Geometry: see drawing. Coordinates: mm, zero at the bounding-box minimum. Give positions to 0.01 mm unless a question says otherwise; leave off trailing zeros.
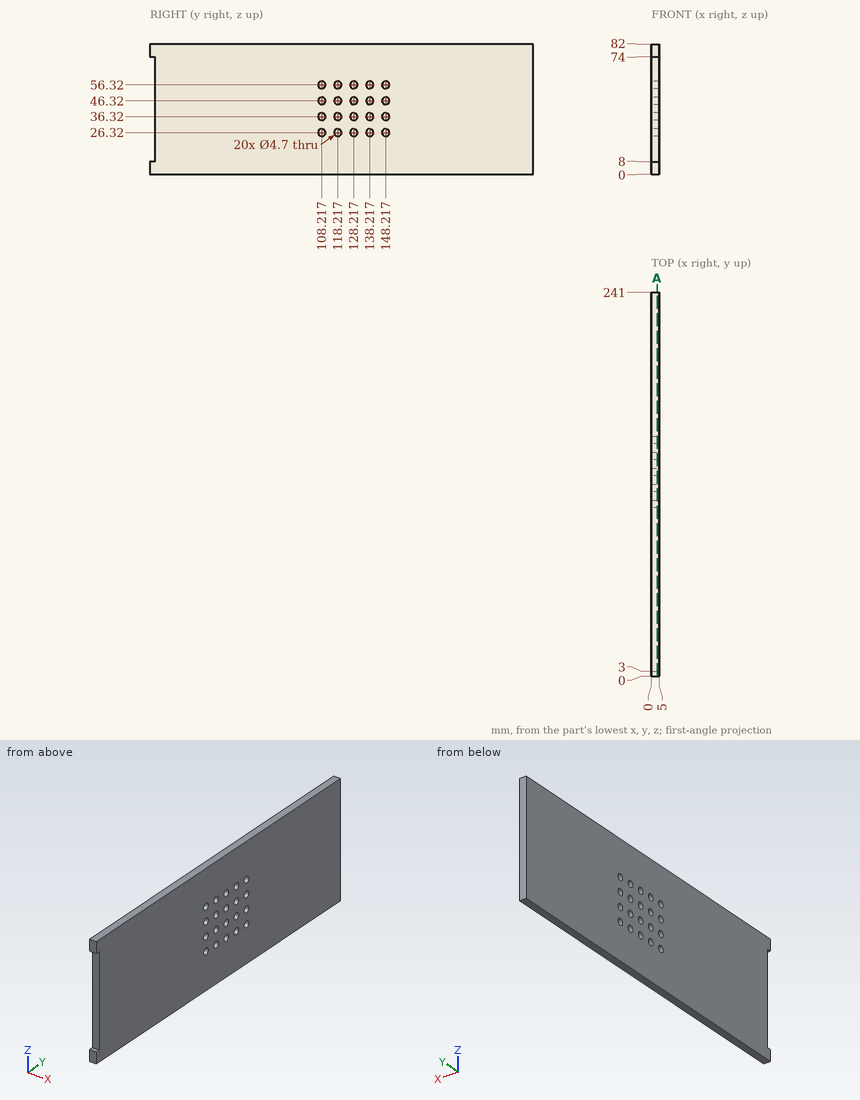
Q1. Pin query (flat end, axial travel): pin 1 (4 mm diameter, centred on y = 128.22, z = 46.32, fed in from +X); pin 2 (2 mm diameter, centred on x = 3.5, z = 36, fed in from -Y). Return the tip coordinate at first contact, or that it passes through.
Q2. Material intervals for line 1 along Y through (x, z) = (1.6, 25); line 2 along Y through (x, z) = (1, 11), sorted ascending.
Q3. Section A-A, the plane x = 3.7. Give the number of separate pieces and of enclosed holes in the cut face, then the cut area to 3 significant figures.
Solutions:
1. pin 1: passes through
1. pin 2: stops at y = 3
2. line 1: y = 3 to 106.27, 110.16 to 116.27, 120.16 to 126.27, 130.16 to 136.27, 140.16 to 146.27, 150.16 to 241
2. line 2: y = 3 to 241
3. separate pieces: 1
3. enclosed holes: 20
3. area: 19,200 mm2
